Could you check a few things on this model? Use its own coordinates, in mm. A direction names the side the tool comes from. Round coordinates to 2 decimals unless told otherwise and drop trailing zeros. Loops run counter-clockwise (first coordinate to the right, second up) from the corner with the lowest first, then second, coordinate; pieces in that order, holes last.
from build123d import *

# Parameters (mm, degrees)
F0_R     = 23.114
F1_DEPTH = 4.699
F2_R     = 1.27
F3_R     = 13.335
F3_R_2   = 12.7
F4_DEPTH = 3.175


with BuildPart() as f1:
    # F0 (on Top) → F1 (new body)
    with BuildSketch(Plane.XY):
        Circle(F0_R)
    extrude(amount=-F1_DEPTH)

    # F2
    f2_edges = [f1.edges().sort_by_distance(p)[0] for p in [
        (-23.114, 0, 0),
    ]]
    fillet(f2_edges, radius=F2_R)

    # F3 (on face) → F4 (cut)
    with BuildSketch(Plane.XY):
        Circle(F3_R)
        Circle(F3_R_2, mode=Mode.SUBTRACT)
    extrude(amount=-F4_DEPTH, mode=Mode.SUBTRACT)


solid = f1.part
Item 1: If we section it at C-C, the plane z = -4: Please give me the cut outline in (x, y).
Results list:
outline: circle Ø46.23 at (0, 0)
Item 2: Will these pins go through, and if not, where does the flat tip stop? pin 1 (1.5 mm diameter, centred on y = -3, z = -2, fed in from +X); pin 2 (6 mm diameter, centred on x = -5, y = -7, fed in from +Z).
Results list:
pin 1: stops at x = 23
pin 2: stops at z = 0
Item 3: We'd pull the mould along X, two halves only. Please class faces 3 (the flat face through (0, 0, -4.699)), 4 (the cylindrical face through (12.426, 19.49, -2.96)), 5 (the cylindrical face through (-2.75, -12.4, -1.57)): released by +X, released by -X, zero draft, split by the parting line, or undercut.
Results list:
face 3: zero draft
face 4: split by the parting line
face 5: undercut
Item 4: If we section it at A-A, the plane y = 0: Please give me the cut outline in (x, z) (3 decimals), then the cut area to 3 significant figures.
Results list:
outline: (-23.114, -4.699) - (23.114, -4.699) - (23.114, -1.27) arc R1.27 ccw to (21.844, 0) - (13.335, 0) - (13.335, -3.175) - (12.7, -3.175) - (12.7, 0) - (-12.7, 0) - (-12.7, -3.175) - (-13.335, -3.175) - (-13.335, 0) - (-21.844, 0) arc R1.27 ccw to (-23.114, -1.27) - close
area: 213 mm2
Item 5: For faces 1 (the flat face through (0, 0, 0)), 2 (the flat face through (12, -5, -3.175)), which set-ups out of +Z, -Z, +X, -X, +Y, -Y let a thin tool reach every point of the face, with its end or its side?
Results list:
face 1: +Z, +X, -X, +Y, -Y
face 2: +Z
Item 6: If I drill on line 1 along Y through (x, z) = (0, -2.2) (3 decimals); line 2 along X through (y, z) = (3, -2.3); line 3 along Y through (x, z) = (8.5, -0.8), over which ranges is the centre line in solid material (lowest first)?
Results list:
line 1: y = -23.114 to -13.335, -12.7 to 12.7, 13.335 to 23.114
line 2: x = -22.92 to -12.99, -12.34 to 12.34, 12.99 to 22.92
line 3: y = -21.4 to -10.27, -9.44 to 9.44, 10.27 to 21.4
